```python
from build123d import *

# Parameters (mm, degrees)
F0_W           = 20.32
F0_H           = 91.44
F1_DEPTH       = 12.7
F3_D           = 6.35
F3_CBORE_D     = 10.922
F3_CBORE_DEPTH = 6.35


with BuildPart() as f1:
    # F0 (on Top) → F1 (new body)
    with BuildSketch(Plane.XY):
        Rectangle(F0_W, F0_H)
    extrude(amount=F1_DEPTH)

    # F3 (through all)
    with Locations(Plane.XY.offset(12.7)):
        with Locations((0, 15.24), (0, -15.24)):
            CounterBoreHole(F3_D / 2, F3_CBORE_D / 2, F3_CBORE_DEPTH)


solid = f1.part
```
Build history of the part. All positions in model axes, mm. A direction names the side the tool comes from. Round coordinates to 2 decimals unless told otherwise and drop trailing zeros. Loops run counter-clockwise (first coordinate to the right, second up) from the corner with the lowest first, then second, coordinate; pieces in that order, holes last.
Item 1: Pin check, flat tip, straight feed: P1, Ø5, axis at x = 0, y = 15.24, coming from the +Z side. Stop position of the tip, or through.
Item 2: Saw through at B-B (x = 0). List the corners of the cut face in (y, z) (3 decimals), then the cut area to 3 significant figures.
Item 3: Saw through at A-A (y = 15.24). List the corners of the cut face in (x, z) (3 decimals).
Item 4: Two-plate mould, pull along Y, no slides. Class faces 3 (the face through (0, -45.72, 6)), 4 (the face through (0, 1, 12.7)), 5 (the face through (0.69, 12.14, 3.13)): released by +Y, released by -Y, zero draft, split by the parting line, or undercut.
Item 5: Saw through at C-C (z = 10.5). List the corners of the cut face in (x, y), then the cut area to 3 significant figures.
Item 6: Drill centre lines: line 1 along Y through (x, z) = (0, 9.25); line 2 along Y through (x, z) = (0, 4) (3 decimals); line 3 along X through (y, z) = (18, 9.25). Where is each one in solid material? Low to high.
Item 7: Saw through at D-D (x = 4.25). List the corners of the cut face in (y, z).
Item 8: Which spindle directions (+Z, -Z, +X, -X, +Y, -Y) get a long thin tool onto all of the face, cutting with end or side? Do faces 1 (the face through (2, -18, 6.35)), 2 (the face through (10.16, -1, 6)). Say none if no direction does.
Worked answers:
1. P1: passes through
2. outline: (-45.72, 0) - (-18.415, 0) - (-18.415, 6.35) - (-20.701, 6.35) - (-20.701, 12.7) - (-45.72, 12.7) - close; (-12.065, 0) - (12.065, 0) - (12.065, 6.35) - (9.779, 6.35) - (9.779, 12.7) - (-9.779, 12.7) - (-9.779, 6.35) - (-12.065, 6.35) - close; (18.415, 0) - (45.72, 0) - (45.72, 12.7) - (20.701, 12.7) - (20.701, 6.35) - (18.415, 6.35) - close
2. area: 942 mm2
3. outline: (-10.16, 0) - (-3.175, 0) - (-3.175, 6.35) - (-5.461, 6.35) - (-5.461, 12.7) - (-10.16, 12.7) - close; (3.175, 0) - (10.16, 0) - (10.16, 12.7) - (5.461, 12.7) - (5.461, 6.35) - (3.175, 6.35) - close
4. face 3: released by -Y
4. face 4: zero draft
4. face 5: undercut
5. outline: (-10.16, -45.72) - (10.16, -45.72) - (10.16, 45.72) - (-10.16, 45.72) - close; hole circle Ø10.92 at (0, -15.24); hole circle Ø10.92 at (0, 15.24)
5. area: 1,670 mm2
6. line 1: y = -45.72 to -20.7, -9.78 to 9.78, 20.7 to 45.72
6. line 2: y = -45.72 to -18.415, -12.065 to 12.065, 18.415 to 45.72
6. line 3: x = -10.16 to -4.71, 4.71 to 10.16
7. outline: (-45.72, 0) - (45.72, 0) - (45.72, 12.7) - (18.67, 12.7) - (18.67, 6.35) - (11.81, 6.35) - (11.81, 12.7) - (-11.81, 12.7) - (-11.81, 6.35) - (-18.67, 6.35) - (-18.67, 12.7) - (-45.72, 12.7) - close
8. face 1: +Z
8. face 2: +Z, -Z, +X, +Y, -Y
